from build123d import *

# Parameters (mm, degrees)
SKETCH1_R             = 1.5
SKETCH1_R_2           = 12.5
BOSS_EXTRUDE1_DEPTH   = 5
BODY_MOVE_COPY1_ANGLE = 119.711745949


with BuildPart() as part:
    # Sketch1 → Boss-Extrude1 (new body)
    with BuildSketch(Plane(origin=(0, 0, 0), x_dir=(1, 0, 0), z_dir=(0, 1, 0))):
        with BuildLine():
            Line((-75, -75), (65, -75))
            ThreePointArc((65, -75), (72.071067812, -72.071067812), (75, -65))
            Line((75, -65), (75, 65))
            ThreePointArc((75, 65), (72.071067812, 72.071067812), (65, 75))
            Line((65, 75), (-75, 75))
            Line((-75, 75), (-97.913420794, 18.506857518))
            ThreePointArc((-97.913420794, 18.506857518), (-98.351985938, 17.031769181), (-98.5, 15.5))
            Line((-98.5, 15.5), (-98.5, -15.5))
            ThreePointArc((-98.5, -15.5), (-98.351985938, -17.031769181), (-97.913420794, -18.506857518))
            Line((-97.913420794, -18.506857518), (-75, -75))
        make_face()
        with Locations(Location((-90.5, 15.5, 0), (0, 0, 270))):
            Circle(SKETCH1_R, mode=Mode.SUBTRACT)
        with Locations(Location((-90.5, -15.5, 0), (0, 0, 270))):
            Circle(SKETCH1_R, mode=Mode.SUBTRACT)
        with Locations(Location((-59.5, -15.5, 0), (0, 0, 270))):
            Circle(SKETCH1_R, mode=Mode.SUBTRACT)
        with Locations(Location((-59.5, 15.5, 0), (0, 0, 270))):
            Circle(SKETCH1_R, mode=Mode.SUBTRACT)
        with Locations(Location((-75, 0, 0), (0, 0, 270))):
            Circle(SKETCH1_R_2, mode=Mode.SUBTRACT)
        with Locations(Location((-65, 65, 0), (0, 0, 270))):
            Circle(SKETCH1_R, mode=Mode.SUBTRACT)
        with Locations(Location((65, 65, 0), (0, 0, 270))):
            Circle(SKETCH1_R, mode=Mode.SUBTRACT)
        with Locations(Location((65, -65, 0), (0, 0, 270))):
            Circle(SKETCH1_R, mode=Mode.SUBTRACT)
        with Locations(Location((-65, -65, 0), (0, 0, 270))):
            Circle(SKETCH1_R, mode=Mode.SUBTRACT)
        with Locations(Location((0, 0, 0), (0, 0, 270))):
            Circle(SKETCH1_R, mode=Mode.SUBTRACT)
    extrude(amount=BOSS_EXTRUDE1_DEPTH)


with BuildPart() as part_1:
    # Body-Move/Copy1: moved
    add(part.part.moved(Location((0, 0, 0))).rotate(Axis((-6.951895858, -2.256414426, 4.756414426), (-0.5807091426084982, 0.5756634831611324, -0.5756634831615567)), BODY_MOVE_COPY1_ANGLE))


with BuildPart() as part_2:
    # Body-Move/Copy2: moved
    add(part_1.part.moved(Location((11.64746321, 9.2495526, 0))))


solid = part_2.part
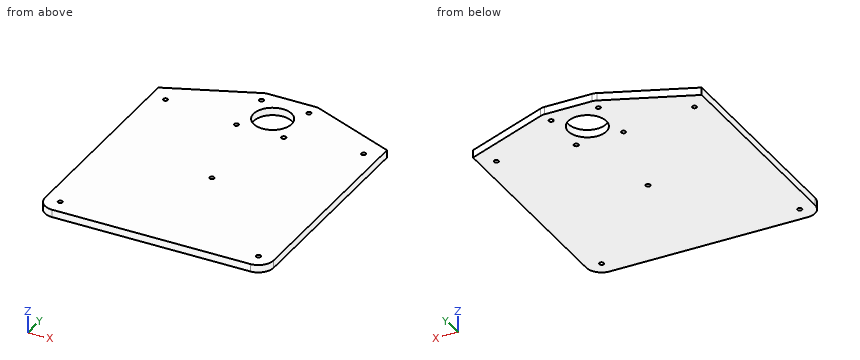
Could you check a few things on this model? Use its own coordinates, in mm. Give positions to 0.01 mm unless a question says otherwise; leave off trailing zeros. Loops run counter-clockwise (first coordinate to the right, second up) from the corner with the lowest first, then second, coordinate; pieces in that order, holes last. Notation, with made-up numbers: (69.25, -9.5) -> (121.25, -9.5) arc R12 ccw to (121.25, 4.5) -> close; hole circle Ø2 at (-37.5, 50). An arc over 180 degrees is marked (long way). Answer as CSV lines item,"result". Start each with the question number.
(1) If we section it at C-C on x = -28: Write out the boundary of the cut face in (y, z).
(2) I'm going to push flat-ended pins straight in: pin 1 Ø3 at (y, z) = (42, 2) entering from -X; pin 2 Ø1.5 at (x, z) = (23.5, 1) entering from -Y. Where does each tip first touch, or does it pass through?
(3) I need wall thicknesses on probe 1 along X at (y, z) = (0, 0.2); probe 2 along X at (y, z) = (68.5, 1.6); probe 3 along Y at (x, z) = (4.5, -0.15). Which ranges of each line are inside material? Lowest first, please.
(4) If we section it at D-D on x = 42: Write out the boundary of the cut face in (y, z).
(5) If we section it at B-B on x = 5: Write out the boundary of the cut face in (y, z), then the cut area to 3 significant figures.
(6) If we section it at A-A on z = 1.55: Count the separate pieces of the cut face and the enclosed holes in it, then the cut area to 3 significant figures.
Computed:
1,outline,"(-75.25, -2.5) -> (94.16, -2.5) -> (94.16, 2.5) -> (-75.25, 2.5) -> close"
2,pin 1,"stops at x = -75.38"
2,pin 2,"stops at y = -74.8"
3,probe 1,"x = -75 to -1.5, 1.5 to 75"
3,probe 2,"x = -75.6 to -11.33, 10.02 to 74.41"
3,probe 3,"y = -74.96 to 63.61, 86.38 to 98.54"
4,outline,"(-74.64, -2.5) -> (88.44, -2.5) -> (88.44, 2.5) -> (-74.64, 2.5) -> close"
5,outline,"(-74.96, -2.5) -> (63.85, -2.5) -> (63.85, 2.5) -> (-74.96, 2.5) -> close; (86.15, -2.5) -> (98.55, -2.5) -> (98.55, 2.5) -> (86.15, 2.5) -> close"
5,area,"756 mm2"
6,separate pieces,"1"
6,enclosed holes,"10"
6,area,"24,100 mm2"
